Geometry: final body of the model. Coordinates: model frame, mm. Face numbers are marked on the shaded views. A direction names the side the tool comes from. Round coordinates to 2 decimals unless told otherwise and drop trailing zeros. Loops run counter-clockwise (first coordinate to the right, second up) from the corner with the lowest first, then second, coordinate; pieces in that order, holes last. Notation, with made-up numbers: (8.25, -6) - (23.25, -6) arc R10 cw to (23.25, 6) - close; hole circle Ø8 at (-38, 71). An arc over 180 degrees is marked (long way). Answer as a JSON object with one key per item and string values. Group by question number.
Item 1: First-contact query: pin 1 (4 mm diameter, centred on y = 11, z = -21.5, fed in from -X); pin 2 (2 mm diameter, centred on x = -60, y = 9.5, fed in from +Z); pin 3 (2 mm diameter, centred on y = 7, z = 28, fed in from -X) (3 decimals); pin 4 (0.6 mm diameter, centred on x = 35.5, y = 7, fed in from -Z). Flat tips, straight axial feed; report the tip coordinate or a pass-through.
Item 2: Section A-A (z = -23). Return the cut outline in (x, y).
Item 3: Reachability of the marked faces 3 and 4 from +Z, -Z, +X, -X, +Y, -Y: full face, straight path, thin tool, end or side. Return the list, or none.
Item 4: Section B-B (x = -100). Return the cut outline in (y, z), plus the area to 3 significant figures.
Item 5: Line query: line 1 (Z direction, x = 17, y = 17); line 2 (Z direction, x = -72.5, y = 5.75); line 3 (X direction, y = 15.25, z = -2). Output: solid intervals per line, ascending.
Item 6: Draft query along Z for the marked faces 1 and 2. Return one class per face: released by +Z, released by -Z, zero draft, split by the parting line, or undercut.
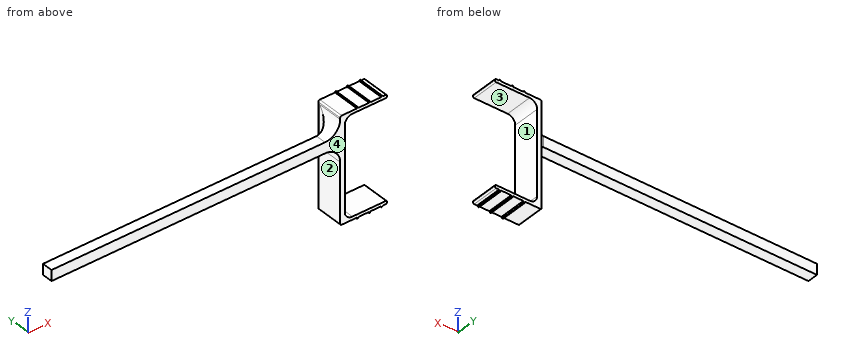
```python
from build123d import *

# Parameters (mm, degrees)
BOSS_EXTRUDE1_DEPTH = 18
FILLET1_R           = 5
FILLET2_R           = 1
SKETCH1_3_W         = 190
SKETCH1_3_H         = 7
BOSS_EXTRUDE2_DEPTH = 7
FILLET3_R           = 10


with BuildPart() as part:
    # Sketch1 → Boss-Extrude1 (new body)
    with BuildSketch(Plane(origin=(0, 0, 0), x_dir=(1, 0, 0), z_dir=(0, 1, 0))):
        with BuildLine():
            ThreePointArc((37.053352185, -32.5), (37.61903761, -32.734314575), (37.853352185, -33.3))
            Line((37.853352185, -33.3), (37.853352185, -33.7))
            ThreePointArc((37.853352185, -33.7), (37.61903761, -34.265685425), (37.053352185, -34.5))
            Line((37.053352185, -34.5), (35.151371079, -34.5))
            Line((35.151371079, -34.5), (34.651371079, -35.2))
            Line((34.651371079, -35.2), (34.053352185, -35.2))
            Line((34.053352185, -35.2), (34.053352185, -34.5))
            Line((34.053352185, -34.5), (27.151371079, -34.5))
            Line((27.151371079, -34.5), (26.651371079, -35.2))
            Line((26.651371079, -35.2), (26.053352185, -35.2))
            Line((26.053352185, -35.2), (26.053352185, -34.5))
            Line((26.053352185, -34.5), (19.151371079, -34.5))
            Line((19.151371079, -34.5), (18.651371079, -35.2))
            Line((18.651371079, -35.2), (18.053352185, -35.2))
            Line((18.053352185, -35.2), (18.053352185, -34.5))
            Line((18.053352185, -34.5), (7.053352185, -34.5))
            Line((7.053352185, -34.5), (7.053352185, 0))
            Line((7.053352185, 0), (10.053352185, 0))
            Line((10.053352185, 0), (10.053352185, -32.5))
            Line((10.053352185, -32.5), (37.053352185, -32.5))
        make_face()
    extrude(amount=BOSS_EXTRUDE1_DEPTH)

    # Fillet1
    fillet1_edges = [part.edges().sort_by_distance(p)[0] for p in [
        (10.053352185, 9, 32.5),
    ]]
    fillet(fillet1_edges, radius=FILLET1_R)

    # Fillet2
    fillet2_edges = [part.edges().sort_by_distance(p)[0] for p in [
        (7.053352185, 9, 34.5),
    ]]
    fillet(fillet2_edges, radius=FILLET2_R)

    # Mirror1: part across plane


with BuildPart() as part_1:
    add(part.part)
    add(part.part.mirror(Plane(origin=(0, 18, 0), x_dir=(1, 0, 0), z_dir=(0, 0, -1))))

    # Sketch1_3 → Boss-Extrude2 (add)
    with BuildSketch(Plane(origin=(0, 0, 0), x_dir=(1, 0, 0), z_dir=(0, 1, 0))):
        with Locations((-87.946647815, -19)):
            Rectangle(SKETCH1_3_W, SKETCH1_3_H)
    extrude(amount=BOSS_EXTRUDE2_DEPTH)

    # Fillet3
    fillet3_edges = [part_1.edges().sort_by_distance(p)[0] for p in [
        (7.053352185, 7, 19),
        (7.053352185, 3.5, 22.5),
        (7.053352185, 3.5, 15.5),
    ]]
    fillet(fillet3_edges, radius=FILLET3_R)


solid = part_1.part
```
Values:
{
 "1": {"pin 1": "stops at x = 7.05", "pin 2": "passes through", "pin 3": "stops at x = 5.405", "pin 4": "stops at z = -34.5"},
 "2": {"outline": "(7.05, 0) - (10.05, 0) - (10.05, 18) - (7.05, 18) - close"},
 "3": {"face 3": "+X, +Y, -Y", "face 4": "+Z, -Z, +X, -X, -Y"},
 "4": {"outline": "(0, 15.5) - (7, 15.5) - (7, 22.5) - (0, 22.5) - close", "area": "49.0 mm^2"},
 "5": {"line 1": "z = -34.5 to -32.5, 32.5 to 34.5", "line 2": "z = 15.5 to 22.5", "line 3": "x = 7.05 to 10.05"},
 "6": {"face 1": "undercut", "face 2": "zero draft"}
}
